from build123d import *

# Parameters (mm, degrees)
BOSS_EXTRUDE2_DEPTH = 600
SKETCH2_W           = 179.507885947
SKETCH2_H           = 0.1
BOSS_EXTRUDE3_DEPTH = 10
SKETCH3_W           = 179.507885947
SKETCH3_H           = 0.1
BOSS_EXTRUDE4_DEPTH = 10


with BuildPart() as part:
    # Sketch1 → Boss-Extrude2 (new body)
    with BuildSketch(Plane.XY):
        Polygon((-1723.971070815, 565.254300802), (-1544.645451435, 573.341534617), (-1544.649956659, 573.44143308), (-1723.97557604, 565.354199265), align=None)
    extrude(amount=BOSS_EXTRUDE2_DEPTH)

    # Sketch2 → Boss-Extrude3 (add)
    with BuildSketch(Plane(origin=(-28.943777696, 641.796809779, 0), x_dir=(0.998984632, 0.045052248, 0), z_dir=(-0.045052248, 0.998984632, 0))):
        with Locations((-1607.000685751, -0.05)):
            Rectangle(SKETCH2_W, SKETCH2_H)
    extrude(amount=-BOSS_EXTRUDE3_DEPTH)

    # Sketch3 → Boss-Extrude4 (add)
    with BuildSketch(Plane(origin=(-28.943777696, 641.796809779, 0), x_dir=(0.998984632, 0.045052248, 0), z_dir=(-0.045052248, 0.998984632, 0))):
        with Locations((-1607.000685751, -599.95)):
            Rectangle(SKETCH3_W, SKETCH3_H)
    extrude(amount=-BOSS_EXTRUDE4_DEPTH)


solid = part.part
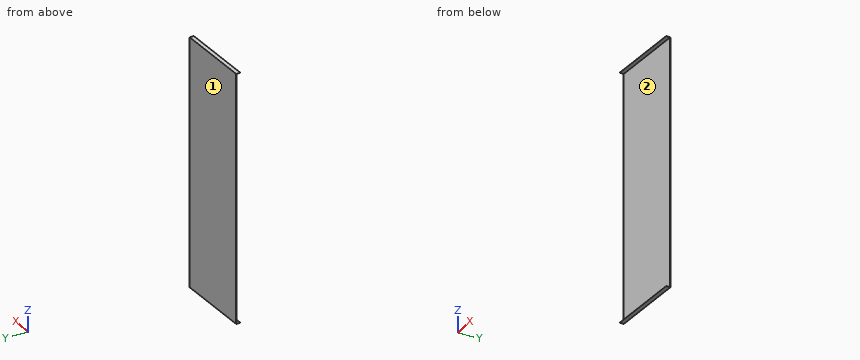
The listing builds one solid part. Answer for the finished solid, in the listing's coordinates (mm). Face numbers are marked on the shaded views. Give positions to 0.01 mm unless a question says otherwise; leave off trailing zeros. Write each loop counter-clockwise with the first axis right and the second up, starting at its lowest first coordinate (ties: lowest second). Pieces come first, ordered by that corner, then holes.
Item 1: Section A-A, the plane y = 558.5 is taken. Write down the section's boundary in (x, z), plus the area to 3 significant figures.
Item 2: Section C-C, the plane z = 104.5 is taken. Write down the section's boundary in (x, y), plus the area to 3 significant figures.
Item 3: Determine the mould class of the marked faces 1 and 2 for opening direction Z: released by +Z, released by -Z, zero draft, split by the parting line, or undercut.
Item 4: Flat-ended cylindrical pins translate along their axes: P1, Ø3, axis at x = -1569.5, z = 506.5, coming from the +Y side; P2, Ø1, axis at x = -1615.5, z = 432.5, coming from the -Y side. Find the tip coordinate at first contact, or state that the pin passes through.
Item 5: Section B-B, the plane x = -1618 is taken. Write down the section's boundary in (y, z), plus the area to 3 significant figures.
Completed:
1. outline: (-1723.67, 0) - (-1654, 0) - (-1654, 0.1) - (-1723.67, 0.1) - close; (-1723.67, 599.9) - (-1654, 599.9) - (-1654, 600) - (-1723.67, 600) - close
1. area: 13.9 mm2
2. outline: (-1723.98, 565.35) - (-1723.97, 565.25) - (-1544.65, 573.34) - (-1544.65, 573.44) - close
2. area: 18.0 mm2
3. face 1: zero draft
3. face 2: undercut
4. P1: stops at y = 572.39
4. P2: stops at y = 570.12
5. outline: (560.12, 0) - (570.13, 0) - (570.13, 600) - (560.12, 600) - (560.12, 599.9) - (570.03, 599.9) - (570.03, 0.1) - (560.12, 0.1) - close
5. area: 62.0 mm2
